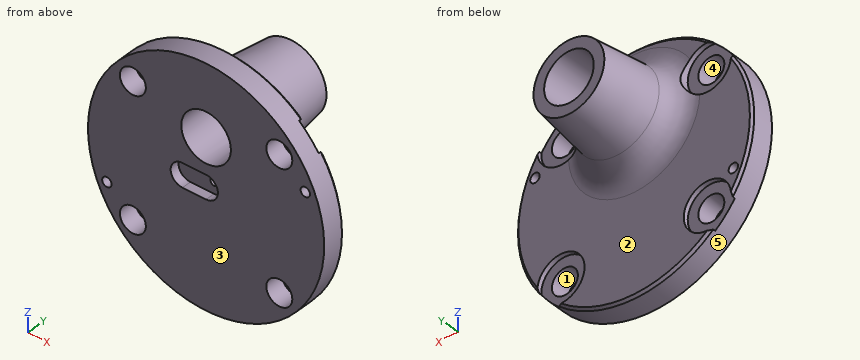
from build123d import *

# Parameters (mm, degrees)
SKETCH_1_R               = 50
EXTRUDE_1_DEPTH          = 10
FILLET_1_R               = 10
F_1_UN_DEPTH             = 79.0320447
F_1_UN_DEPTH_BACK        = 2
SKETCH_2_R               = 10
SKETCH_2_R_2             = 5.5
CUT_EXTRUDE_3_DEPTH      = 79.0320447
CUT_EXTRUDE_3_DEPTH_BACK = 79.0320447
SKETCH_2_3_R             = 5.5
SKETCH_6_R               = 10.5
CUT_EXTRUDE_4_DEPTH      = 83.758685345
SKETCH_7_R               = 2
CUT_EXTRUDE_6_DEPTH      = 83.758685345
CUT_EXTRUDE_7_DEPTH      = 4
SWEEP_1_OUTLINE_W        = 1.5
SWEEP_1_OUTLINE_H        = 22.476650491
CHAMFER_2_SIZE           = 1


# Read off the part's stored shape, not the designer's step: 切除-扫描1
with BuildPart() as part:
    # 草图1 → 凸台-拉伸1 (new body)
    with BuildSketch(Plane(origin=(0, 0, 0), x_dir=(1, 0, 0), z_dir=(0, 1, 0))):
        with Locations(Location((0, 0, 0), (0, 0, 270))):
            Circle(SKETCH_1_R)
    extrude(amount=EXTRUDE_1_DEPTH)

    # 草图5 → 旋转1 (revolve)
    with BuildSketch(Plane(origin=(0, 0, 0), x_dir=(0, 0, -1), z_dir=(1, 0, 0))):
        Polygon((-20, 10), (-20, 43), (-35, 43), (-39, 10), align=None)
    revolve(axis=Axis((0, 37.278151035, 20), (0, -1, 0)))

    # 圆角1
    fillet_1_edges = [part.edges().sort_by_distance(p)[0] for p in [
        (0, 10, 1),
    ]]
    fillet(fillet_1_edges, radius=FILLET_1_R)

    # 草图2 → 切除-拉伸1 un (cut, two sides: drawn at the far end of the back side and taken through both)
    # profile 1 of 4: a face of its own
    with BuildSketch(Plane(origin=(0, 10, 0), x_dir=(1, 0, 0), z_dir=(0, 1, 0)).offset(-F_1_UN_DEPTH_BACK)):
        with Locations((31, 28)):
            Circle(SKETCH_2_R)
        with Locations(Location((31, 28, 0), (0, 0, 270))):
            Circle(SKETCH_2_R_2, mode=Mode.SUBTRACT)
    # profile 2 of 4: a face of its own
    with BuildSketch(Plane(origin=(0, 10, 0), x_dir=(1, 0, 0), z_dir=(0, 1, 0)).offset(-F_1_UN_DEPTH_BACK)):
        with Locations((-31, 28)):
            Circle(SKETCH_2_R)
        with Locations(Location((-31, 28, 0), (0, 0, 90))):
            Circle(SKETCH_2_R_2, mode=Mode.SUBTRACT)
    # profile 3 of 4: a face of its own
    with BuildSketch(Plane(origin=(0, 10, 0), x_dir=(1, 0, 0), z_dir=(0, 1, 0)).offset(-F_1_UN_DEPTH_BACK)):
        with Locations((-31, -28)):
            Circle(SKETCH_2_R)
        with Locations(Location((-31, -28, 0), (0, 0, 52.073353544))):
            Circle(SKETCH_2_R_2, mode=Mode.SUBTRACT)
    # profile 4 of 4: a face of its own
    with BuildSketch(Plane(origin=(0, 10, 0), x_dir=(1, 0, 0), z_dir=(0, 1, 0)).offset(-F_1_UN_DEPTH_BACK)):
        with Locations((31, -28)):
            Circle(SKETCH_2_R)
        with Locations(Location((31, -28, 0), (0, 0, 90))):
            Circle(SKETCH_2_R_2, mode=Mode.SUBTRACT)
    extrude(amount=F_1_UN_DEPTH + F_1_UN_DEPTH_BACK, mode=Mode.SUBTRACT)

    # 草图2<3> → 切除-拉伸3 (cut, two sides: drawn at the far end of the back side and taken through both)
    with BuildSketch(Plane(origin=(0, 10, 0), x_dir=(1, 0, 0), z_dir=(0, 1, 0)).offset(-CUT_EXTRUDE_3_DEPTH_BACK)):
        with Locations(Location((31, 28, 0), (0, 0, 270))):
            Circle(SKETCH_2_3_R)
        with Locations(Location((-31, 28, 0), (0, 0, 270))):
            Circle(SKETCH_2_3_R)
        with Locations(Location((-31, -28, 0), (0, 0, 270))):
            Circle(SKETCH_2_3_R)
        with Locations(Location((31, -28, 0), (0, 0, 270))):
            Circle(SKETCH_2_3_R)
    extrude(amount=CUT_EXTRUDE_3_DEPTH + CUT_EXTRUDE_3_DEPTH_BACK, mode=Mode.SUBTRACT)

    # 草图6 → 切除-拉伸4 (cut, through all)
    with BuildSketch(Plane(origin=(0, 43, 0), x_dir=(1, 0, 0), z_dir=(0, 1, 0))):
        with Locations(Location((0, -20, 0), (0, 0, 270))):
            Circle(SKETCH_6_R)
    extrude(amount=-CUT_EXTRUDE_4_DEPTH, mode=Mode.SUBTRACT)

    # 草图7 → 切除-拉伸6 (cut, through all)
    with BuildSketch(Plane(origin=(0, 0, 0), x_dir=(1, 0, 0), z_dir=(0, 1, 0))):
        with Locations(Location((42, -18, 0), (0, 0, 270))):
            Circle(SKETCH_7_R)
        with Locations(Location((-42, 18, 0), (0, 0, 270))):
            Circle(SKETCH_7_R)
    extrude(amount=CUT_EXTRUDE_6_DEPTH, mode=Mode.SUBTRACT)

    # 草图8 → 切除-拉伸7 (cut)
    with BuildSketch(Plane.XZ):
        with BuildLine():
            Line((0, -5), (-10, -5))
            ThreePointArc((-10, -5), (-15, 0), (-10, 5))
            Line((-10, 5), (0, 5))
            ThreePointArc((0, 5), (5, 0), (0, -5))
        make_face()
    extrude(amount=-CUT_EXTRUDE_7_DEPTH, mode=Mode.SUBTRACT)

    # 切除-扫描1 outline → 切除-扫描1 (revolve, cut)
    with BuildSketch(Plane(origin=(0, 1, -1.732050808), x_dir=(1, 0, 0), z_dir=(0, -0.5000000000000042, 0.8660254037844363))):
        with Locations((0.75, 13.824548036)):
            Rectangle(SWEEP_1_OUTLINE_W, SWEEP_1_OUTLINE_H)
    revolve(axis=Axis((0, 1, -1.732050808), (0, 0.8660254037844363, 0.5000000000000042)), mode=Mode.SUBTRACT)

    # 倒角2
    chamfer_2_edges = [part.edges().sort_by_distance(p)[0] for p in [
        (50, 10, 0),
        (0, 10, -50),
        (-50, 10, 0),
        (17.420003831, 10, 46.867296343),
    ]]
    chamfer(chamfer_2_edges, length=CHAMFER_2_SIZE)


solid = part.part
Part model, mm, in its own coordinate system. Face numbers are marked on the shaded views. A direction names the side the tool comes from. Coordinates: 2 decimals unless noted, no trailing zeros. Loops run counter-clockwise (first coordinate to the right, second up) from the corner with the lowest first, then second, coordinate; pieces in that order, holes last. Notation, with made-up numbers: M -11,62 L 43,62 A29 ccw 43,97 Z; hole C -33,-21 d3. An arc over 180 degrees is marked long. Use a Markdown table: item, result. Add a question column.
Q1. Which spindle directions (+Z, -Z, +X, -X, +Y, -Y) get a long thin tool onto all of the face, cutting with end or side? Do the marked faces 1 and 2. Say none if no direction does.
Q2. Cut at C-C (y = 37). Write the cut outline in (x, z), and give its area (3 significant figures).
Q3. Mould opens along Z. For the marked faces 3, 4 and 5 say: +Z half, -Z half, draft (parallel to the pull), parting line (faces both ways), or undercut.
Q4. Probe L1, parallel to Z at x = -31, y = 9.1; L2, parallel to X at y = 9.1, z = -28; L3, parallel to Y at x = 25, z = -13. List the from-to ranges inside material, lowest first.
Q5. Cut at B-B (y = 16). Give the number of separate pieces and of enclosed holes in the cut face, and give its area (3 significant figures).
Q6. Pin check, flat tips, straight feed: P1, Ø3, axis at x = -7.5, y = 3, coming from the +Z side; P2, Ø10, axis at x = -31, z = -24.5, coming from the +Y side; P3, Ø1.5, axis at y = 9, z = -32, coming from the -X side. Stop position of each tip, or through.
Q7. Cut at A-A (y = 31). Write the cut outline in (x, z), and give its area (3 significant figures).
Worked out:
| question | item | result |
|---|---|---|
| 1 | face 1 | +Y, -Y |
| 1 | face 2 | -Z, +Y |
| 2 | outline | C 0,20 d31.45; hole C 0,20 d21 |
| 2 | area | 431 mm2 |
| 3 | face 3 | draft |
| 3 | face 4 | undercut |
| 3 | face 5 | parting line |
| 4 | L1 | z = -39.1 to -38, -18 to 18, 38 to 39.1 |
| 4 | L2 | x = -41.3 to -41, -21 to 21, 41 to 41.3 |
| 4 | L3 | y = 0 to 10 |
| 5 | separate pieces | 1 |
| 5 | enclosed holes | 2 |
| 5 | area | 744 mm2 |
| 6 | P1 | stops at z = 49.64 |
| 6 | P2 | stops at y = 8 |
| 6 | P3 | stops at x = -22.2 |
| 7 | outline | C 0,20 d32.91; hole C 0,20 d21 |
| 7 | area | 504 mm2 |
